Read the model definition and answer for the solid it produces. Units are mm, in the model's axes. A direction names the side the tool comes from. Give positions to 0.01 mm unless a question says otherwise; leave off trailing zeros. Write each loop counter-clockwise with the first axis right and the second up, starting at its lowest first coordinate (ties: lowest second). Pieces come first, ordered by that corner, then holes. Notation, with made-up numbers: (23, -29) -> (80, -29) arc R21 ccw to (80, -6) -> close; hole circle Ø11 at (-2.75, 67). An arc over 180 degrees is marked (long way). Answer as CSV lines item,"result". Start each with the question number.
1. A tool of negligible diameter and unlimited length cuts with its end or side. For faces 1 (the flat face through (186.5, 0, 3)), 2 (the flat face through (114, 5, 0)), from which of +Z, -Z, +X, -X, +Y, -Y can it reach the whole face along a straight path? Write none if from no direction.
2. The part is cut by section B-B, the plane z = 4.5. Give the number of separate pieces and of enclosed holes in the cut face, and give its area (3 significant figures).
3. Find the intervals of material crossed by line 1 (Y direction, x = 147, z = 3.5); line 2 (Y direction, x = 0, z = 4.75); line 3 (Y direction, x = 219, z = 1.75), in increasing order.
4. For a pull along Y with two mould halves and no side action, classify faces 3 (the flat face through (63, -4, 3)), 4 (the cylindrical face through (203.623, 7.133, 3.131)), 5 (the flat face through (101, -8, 3)), 6 (the flat face through (231.928, 0, 3)) as pulls with the +Y half, pulls with the -Y half, needs draft (parallel to the pull), parting line crosses it, or undercut.
5. The part is cut by section A-A, the plane x = 110.5. Determine the outline of the cut face in (y, z).
from build123d import *

# Parameters (mm, degrees)
SKETCH1_R           = 1
SKETCH1_R_2         = 3.25
SKETCH1_R_3         = 3.75
BOSS_EXTRUDE1_DEPTH = 6.35


with BuildPart() as part:
    # Sketch1 → Boss-Extrude1 (new body)
    with BuildSketch(Plane(origin=(0, 0, 0), x_dir=(-1, 0, 0), z_dir=(0, 0, -1))):
        with BuildLine():
            Line((0, 8), (-200, 8))
            ThreePointArc((-200, 8), (-203.670651742, 7.108186533), (-206.52291932, 4.631578948))
            ThreePointArc((-206.52291932, 4.631578948), (-207.05771949, 4.167215025), (-207.745966692, 4))
            Line((-207.745966692, 4), (-231.92820323, 4))
            Line((-231.92820323, 4), (-231.92820323, -4))
            Line((-231.92820323, -4), (-207.745966692, -4))
            ThreePointArc((-207.745966692, -4), (-207.05771949, -4.167215025), (-206.52291932, -4.631578947))
            ThreePointArc((-206.52291932, -4.631578947), (-203.670651742, -7.108186533), (-200, -8))
            Line((-200, -8), (0, -8))
            ThreePointArc((0, -8), (8, 0), (0, 8))
        make_face()
        with Locations((-159, 0)):
            Circle(SKETCH1_R, mode=Mode.SUBTRACT)
        with Locations((-184, 0)):
            Circle(SKETCH1_R, mode=Mode.SUBTRACT)
        Circle(SKETCH1_R_2, mode=Mode.SUBTRACT)
        with Locations((-200, 0)):
            Circle(SKETCH1_R_3, mode=Mode.SUBTRACT)
        with Locations((-213.982050808, 0)):
            Circle(SKETCH1_R, mode=Mode.SUBTRACT)
        with Locations((-225.946152423, 0)):
            Circle(SKETCH1_R, mode=Mode.SUBTRACT)
        with BuildLine():
            Line((-186.499999983, 1.999999984), (-186.499999983, -1.999999983))
            ThreePointArc((-186.499999983, -1.999999983), (-187.085786426, -3.414213557), (-188.5, -4))
            Line((-188.5, -4), (-190.83484861, -4))
            ThreePointArc((-190.83484861, -4), (-192.026927731, -3.410465468), (-192.281977777, -2.105263158))
            ThreePointArc((-192.281977777, -2.105263158), (-192, 0), (-192.281977777, 2.105263158))
            ThreePointArc((-192.281977777, 2.105263158), (-192.026927731, 3.410465468), (-190.83484861, 4))
            Line((-190.83484861, 4), (-188.5, 4))
            ThreePointArc((-188.5, 4), (-187.085786426, 3.414213558), (-186.499999983, 1.999999984))
        make_face(mode=Mode.SUBTRACT)
        with BuildLine():
            Line((-181.499999977, -2.000000023), (-181.499999977, 2.000000023))
            ThreePointArc((-181.499999977, 2.000000023), (-180.914213546, 3.414213569), (-179.5, 4))
            Line((-179.5, 4), (-163.5, 4))
            ThreePointArc((-163.5, 4), (-162.085786447, 3.414213567), (-161.500000014, 2.000000014))
            Line((-161.500000014, 2.000000014), (-161.500000014, -2.000000014))
            ThreePointArc((-161.500000014, -2.000000014), (-162.085786447, -3.414213566), (-163.5, -4))
            Line((-163.5, -4), (-179.5, -4))
            ThreePointArc((-179.5, -4), (-180.914213546, -3.414213569), (-181.499999977, -2.000000023))
        make_face(mode=Mode.SUBTRACT)
        with BuildLine():
            Line((-49.998863542, -4), (-77.332575695, -4))
            ThreePointArc((-77.332575695, -4), (-81.332575695, 0), (-77.332575695, 4))
            Line((-77.332575695, 4), (-49.998863542, 4))
            ThreePointArc((-49.998863542, 4), (-45.998863542, 0), (-49.998863542, -4))
        make_face(mode=Mode.SUBTRACT)
        with BuildLine():
            Line((-123.416287847, -4), (-154.5, -4))
            ThreePointArc((-154.5, -4), (-155.914213568, -3.41421356), (-156.500000008, -1.999999992))
            Line((-156.500000008, -1.999999992), (-156.500000008, 1.999999992))
            ThreePointArc((-156.500000008, 1.999999992), (-155.914213568, 3.41421356), (-154.5, 4))
            Line((-154.5, 4), (-123.416287847, 4))
            ThreePointArc((-123.416287847, 4), (-119.416287847, 0), (-123.416287847, -4))
        make_face(mode=Mode.SUBTRACT)
        with BuildLine():
            Line((-113.916287847, 4), (-86.832575695, 4))
            ThreePointArc((-86.832575695, 4), (-82.832575695, 0), (-86.832575695, -4))
            Line((-86.832575695, -4), (-113.916287847, -4))
            ThreePointArc((-113.916287847, -4), (-117.916287847, 0), (-113.916287847, 4))
        make_face(mode=Mode.SUBTRACT)
        with BuildLine():
            Line((-40.498863542, 4), (-9.16515139, 4))
            ThreePointArc((-9.16515139, 4), (-7.973072268, 3.410465468), (-7.718022223, 2.105263158))
            ThreePointArc((-7.718022223, 2.105263158), (-8, 0), (-7.718022223, -2.105263158))
            ThreePointArc((-7.718022223, -2.105263158), (-7.973072268, -3.410465468), (-9.16515139, -4))
            Line((-9.16515139, -4), (-40.498863542, -4))
            ThreePointArc((-40.498863542, -4), (-44.498863542, 0), (-40.498863542, 4))
        make_face(mode=Mode.SUBTRACT)
    extrude(amount=-BOSS_EXTRUDE1_DEPTH)


solid = part.part
Results found:
1,face 1,"+Z, -Z"
1,face 2,"-Z, +X, -X, +Y, -Y"
2,separate pieces,"1"
2,enclosed holes,"12"
2,area,"2,200 mm²"
3,line 1,"y = -8 to -4, 4 to 8"
3,line 2,"y = -8 to -3.25, 3.25 to 8"
3,line 3,"y = -4 to 4"
4,face 3,"undercut"
4,face 4,"pulls with the +Y half"
4,face 5,"pulls with the -Y half"
4,face 6,"needs draft"
5,outline,"(-8, 0) -> (-4, 0) -> (-4, 6.35) -> (-8, 6.35) -> close; (4, 0) -> (8, 0) -> (8, 6.35) -> (4, 6.35) -> close"
